Geometry check sheet. Reference: the model listing, model coordinates, mm. Face numbers are marked on the shaded views. A direction names the side the tool comes from. Give positions to 0.01 mm unless a question says otherwise; leave off trailing zeros. Order: outer loops, then holes, each group sorted by start corner. A loop starts at its lowest first (then second) coordinate and runs counter-clockwise, first axis right, second up. Notation, with made-up numbers: M -0.75,0.25 L 25.25,0.25 A22 cw 25.25,37.25 Z; hole C 47.5,21 d3. An arc over 180 degrees is marked long. Answer as CSV lines item,"result".
from build123d import *

# Parameters (mm, degrees)
REVOLVE1_ANGLE     = 180
FILLET1_SIZE       = 4
FILLET1_SIZE_2     = 2
CHAMFER1_SIZE      = 4
CHAMFER1_SIZE2     = 0.705307923
REVOLVE2_ANGLE     = 180
SKETCH3_R          = 1.5
CUT_EXTRUDE1_DEPTH = 10


with BuildPart() as part:
    # Sketch1 → Revolve1 (revolve)
    with BuildSketch(Plane.XY):
        Polygon((0, -9.5), (0, 2), (-5.5, 2), (-5.5, -3.5), (-10, -3.5), (-10, -9.5), align=None)
    revolve(axis=Axis((0, -14.5, 0), (0, 1, 0)), revolution_arc=REVOLVE1_ANGLE)

    # Fillet1
    # an asymmetric fillet: 4, 2 mm, written as the material it takes off along each edge
    with BuildSketch(Plane(origin=(0, -9.5, 0), x_dir=(-0.5389483633149525, 0, -0.8423388045674578), z_dir=(0.8423388045674578, 0, -0.5389483633149525))) as fillet1_piece_1:
        with BuildLine():
            Bezier((10 - FILLET1_SIZE, 0), (10, 0), (10, FILLET1_SIZE_2), weights=[1, 0.707106781, 1])
            Line((10, FILLET1_SIZE_2), (10, 0))
            Line((10, 0), (10 - FILLET1_SIZE, 0))
        make_face()
    revolve(axis=Axis((0, -9.5, 0), (0, 1, 0)), revolution_arc=294.775843921, mode=Mode.SUBTRACT)

    # Chamfer1
    chamfer1_edges = [part.edges().sort_by_distance(p)[0] for p in [
        (0, -3.5, 10),
    ]]
    chamfer1_side = [part.faces().sort_by_distance(p)[0] for p in [
        (0, -3.5, 5.723606798),
    ]]
    chamfer(chamfer1_edges, length=CHAMFER1_SIZE, length2=CHAMFER1_SIZE2, reference=chamfer1_side[0])


with BuildPart() as body_2:
    # Sketch2 → Revolve2 (revolve)
    with BuildSketch(Plane.XY):
        with BuildLine():
            Line((-5.5, 2), (-10, 2))
            Line((-10, 2), (-12.831859955, 3.064721462))
            Line((-12.831859955, 3.064721462), (-15.01308486, 4.913217144))
            Line((-15.01308486, 4.913217144), (-15.974302614, 6.983532307))
            Line((-15.974302614, 6.983532307), (-19.387891627, 6.983532307))
            Line((-19.387891627, 6.983532307), (-22.387891627, 6.983532307))
            Line((-22.387891627, 6.983532307), (-23.863690319, 1.983532307))
            Line((-23.863690319, 1.983532307), (-14.363690319, 1.983532307))
            ThreePointArc((-14.363690319, 1.983532307), (-10.931862112, -9.525985029), (0, -14.5))
            Line((0, -14.5), (0, -9.5))
            Line((0, -9.5), (-5.99955163, -9.5))
            add(Edge.make_bspline(
                [(-5.99955163, -9.5), (-6.613966051, -9.500022958), (-7.200553434, -9.407759327), (-7.834490948, -9.308048049), (-8.370669156, -9.110794638), (-9.014660015, -8.873878269), (-9.427521538, -8.530743599), (-9.68430445, -8.317327925), (-9.82887241, -8.078117533), (-9.999615313, -7.795596589), (-9.999626359, -7.5)],
                knots=[0, 0, 0, 0.25, 0.25, 0.5, 0.5, 0.75, 0.75, 0.875, 0.875, 1, 1, 1], degree=2))
            Line((-9.999626359, -7.5), (-10, -4.205307923))
            Line((-10, -4.205307923), (-6.14232061, -3.5))
            Line((-6.14232061, -3.5), (-5.5, -3.5))
            Line((-5.5, -3.5), (-5.5, 2))
        make_face()
    revolve(axis=Axis((0, -9.5, 0), (0, 1, 0)), revolution_arc=REVOLVE2_ANGLE)

    # Sketch3 → Cut-Extrude1 (cut)
    with BuildSketch(Plane(origin=(0, 6.983532307, 0), x_dir=(1, 0, 0), z_dir=(0, 1, 0))):
        with Locations(Location((13.564701596, -13.564701596, 0), (0, 0, 270))):
            Circle(SKETCH3_R)
    cut_extrude1 = extrude(amount=-CUT_EXTRUDE1_DEPTH, mode=Mode.SUBTRACT)

    # Mirror1: Cut-Extrude1 across plane
    add(cut_extrude1.mirror(Plane(origin=(0, 0, 0), x_dir=(0, 0, 1), z_dir=(1, 0, 0))), mode=Mode.SUBTRACT)


solid = body_2.part
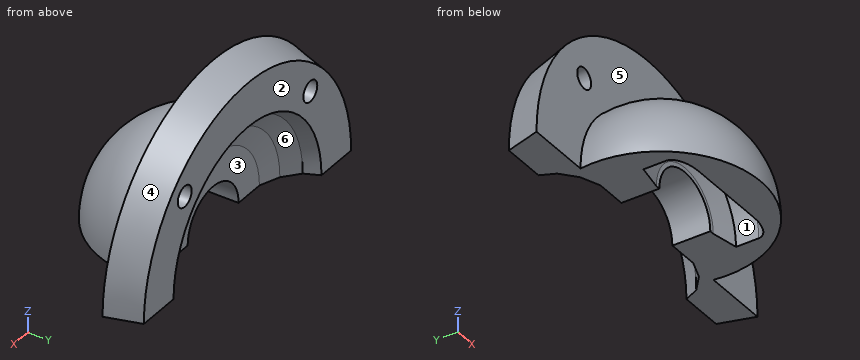
(1) Tool access check on the marked faces 1, 2 and 3. Record the directions out of +Z, -Z, +X, -X, +Y, -Y that give a thin tool (end or side, any length) a straight path to the whole face; none if there is none.
The answers:
face 1,"-Z"
face 2,"+Z, -Z, +X, -X, +Y"
face 3,"-Z, +Y"
(2) Material ranges on line 1 (Y direction, x = 4, z = 20); line 2 (X direction, y = 3.5, z = 9); line 3 (X direction, y = -5.25, z = 6.25), recorded low to high.
The answers:
line 1,"y = 1.98 to 6.98"
line 2,"x = -21.62 to -9.85, 9.85 to 21.62"
line 3,"x = -11.98 to -7.81, 7.81 to 11.98"
(3) Draft check along X on the marked faces 4, 5 and 6. Enter one of: +X half, -X half, draft (parallel to the pull), parting line (faces both ways), or undercut.
The answers:
face 4,"parting line"
face 5,"draft"
face 6,"undercut"
(4) Section check A-A on y = -2. Enter the section's corners in (x, z), then the cut area to 3 significant figures.
The answers:
outline,"M -14.36,0 L -5.5,0 A5.5 cw 5.5,0 L 14.36,0 A14.36 ccw Z"
area,"276 mm2"
(5) Gauge pin test, flat ends, axial feed: P1, Ø8, axis at x = -1.5, z = 5, coming from the +Y side; P2, Ø8, axis at x = 18.5, y = -6, coming from the +Z side; P3, Ø1.5, axis at x = 11, z = 8, coming from the -Y side; P4, Ø7, axis at x = 10.5, z = 12, coming from the -Y side. Record the tip position at first contact, or that the pin passes through.
The answers:
P1,"stops at y = 2"
P2,"passes through"
P3,"stops at y = -6.71"
P4,"stops at y = -7.44"
(6) Section check B-B on y = 1. Enter the section's corners in (x, z), then the cut area to 3 significant figures.
The answers:
outline,"M -14.47,0 L -5.5,0 A5.5 cw 5.5,0 L 14.47,0 A14.47 ccw Z"
area,"281 mm2"
